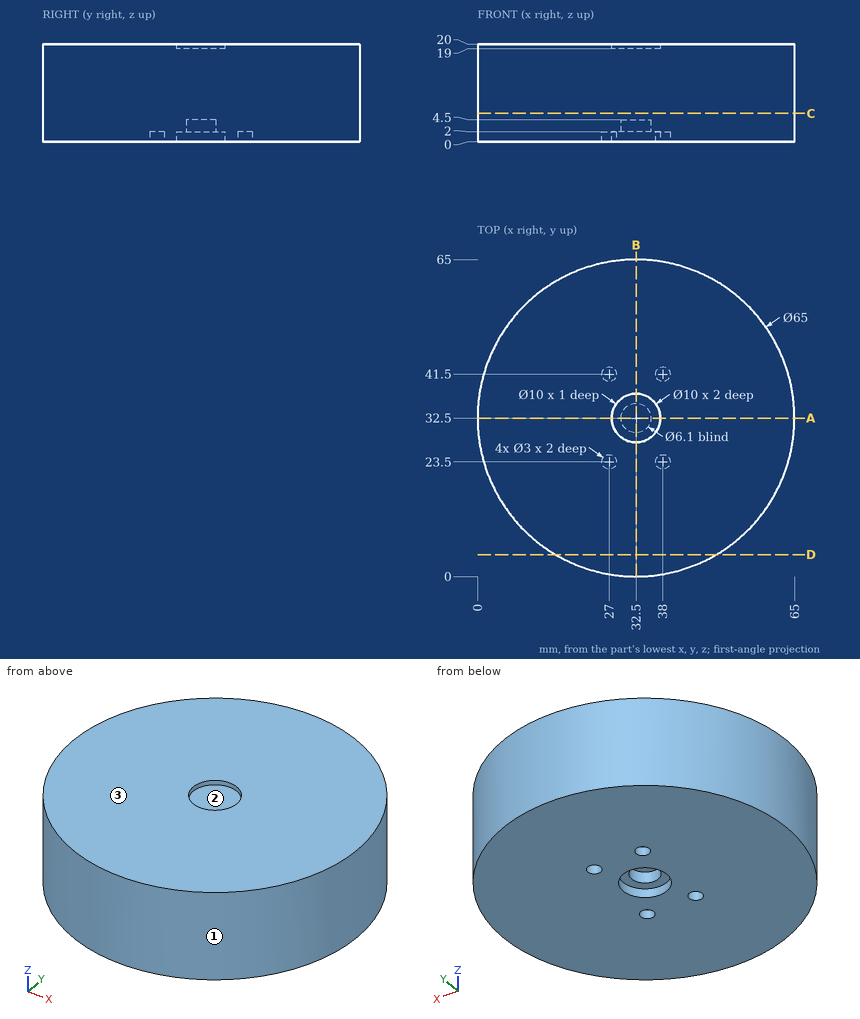
Answer from the drawing. Dimensions are ordinates in mm from the lowest x, y and z of the part. Coordinates: 2 decimals unless noted, no trailing zeros. Write each loop counter-clockwise with the first axis right and the second up, starting at its lowest first coordinate (ties: lowest second). Pieces come first, ordered by that corner, then holes. Notation, with made-up numbers: (46, -18.5) - (96, -18.5) arc R28 ccw to (96, 7.5) - close; hole circle Ø1 at (84.5, 81). An arc over 180 degrees is marked (long way). Return JSON: item names as keys, results as strings.
1. Each of these flat-tipped pins is pushed along its axis until it touches: pin 1 Ø3 at (x, y) = (33, 32.5) entering from -Z; pin 2 Ø8 at (x, y) = (32.5, 32.5) entering from +Z; pin 3 Ø0.9 at (x, y) = (37.5, 23.5) entering from -Z. Where does it stop, or does it pass through?
Final values:
{"pin 1": "z = 4.5", "pin 2": "z = 19", "pin 3": "z = 2"}
2. The part is cut by section A-A on y = 32.5. Determine the outline of the cut face in (x, z), then the cut area to 3 significant figures.
Final values:
{"outline": "(0, 0) - (27.5, 0) - (27.5, 2) - (29.45, 2) - (29.45, 4.5) - (35.55, 4.5) - (35.55, 2) - (37.5, 2) - (37.5, 0) - (65, 0) - (65, 20) - (37.5, 20) - (37.5, 19) - (27.5, 19) - (27.5, 20) - (0, 20) - close", "area": "1,250 mm^2"}
3. The part is cut by section D-D on y = 4.5. Determine the outline of the cut face in (x, z), then the cut area to 3 significant figures.
Final values:
{"outline": "(16, 0) - (49, 0) - (49, 20) - (16, 20) - close", "area": "660 mm^2"}
4. Consider line 1 along Y through (x, z) = (32.5, 19.55); line 2 along Y through (x, z) = (38, 0.6); line 3 along Z through (x, y) = (28, 41). Determine where each line is inside the solid, lowest interval first.
Final values:
{"line 1": "0 to 27.5, 37.5 to 65", "line 2": "0.47 to 22, 25 to 40, 43 to 64.53", "line 3": "2 to 20"}
5. The part is cut by section C-C on z = 5.75. Determine the outline of the cut face in (x, y), then the cut area to 3 significant figures.
Final values:
{"outline": "circle Ø65 at (32.5, 32.5)", "area": "3,320 mm^2"}
6. For a pull along Y with two mould halves and no side action, classify the marked faces 1, 2 and 3 as +Y half, -Y half, draft (parallel to the pull), parting line (faces both ways), or undercut.
Final values:
{"face 1": "parting line", "face 2": "undercut", "face 3": "draft"}
